Build history of the part. All positions in model axes, mm. A direction names the side the tool comes from. Give positions to 0.01 mm unless a question says otherwise; leave off trailing zeros. Write each loop counter-clockwise with the first axis right and the second up, starting at its lowest first coordinate (ties: lowest second). Pieces come first, ordered by that corner, then holes.
from build123d import *

# Parameters (mm, degrees)
ESQUISSE1_W        = 212
ESQUISSE1_H        = 75.3
ESQUISSE1_R        = 2
ESQUISSE1_W_2      = 5
ESQUISSE1_H_2      = 5
BOSS_EXTRU_1_DEPTH = 5


with BuildPart() as part:
    # Esquisse1 → Boss.-Extru.1 (new body)
    with BuildSketch(Plane.XY):
        with Locations((106, 0)):
            Rectangle(ESQUISSE1_W, ESQUISSE1_H)
        with Locations((30, 0)):
            Circle(ESQUISSE1_R, mode=Mode.SUBTRACT)
        with Locations((80, 0)):
            Circle(ESQUISSE1_R, mode=Mode.SUBTRACT)
        with Locations((82, 33.15)):
            Circle(ESQUISSE1_R, mode=Mode.SUBTRACT)
        with Locations((167, 33.15)):
            Circle(ESQUISSE1_R, mode=Mode.SUBTRACT)
        with Locations(Location((167, -33.15, 0), (0, 0, 90))):
            Circle(ESQUISSE1_R, mode=Mode.SUBTRACT)
        with Locations(Location((82, -33.15, 0), (0, 0, 90))):
            Circle(ESQUISSE1_R, mode=Mode.SUBTRACT)
        with Locations((74.5, 33.15)):
            Rectangle(ESQUISSE1_W_2, ESQUISSE1_H_2, mode=Mode.SUBTRACT)
        with Locations((89.5, 33.15)):
            Rectangle(ESQUISSE1_W_2, ESQUISSE1_H_2, mode=Mode.SUBTRACT)
        with Locations((159.5, 33.15)):
            Rectangle(ESQUISSE1_W_2, ESQUISSE1_H_2, mode=Mode.SUBTRACT)
        with Locations((174.5, 33.15)):
            Rectangle(ESQUISSE1_W_2, ESQUISSE1_H_2, mode=Mode.SUBTRACT)
        with Locations((159.5, -33.15)):
            Rectangle(ESQUISSE1_W_2, ESQUISSE1_H_2, mode=Mode.SUBTRACT)
        with Locations((174.5, -33.15)):
            Rectangle(ESQUISSE1_W_2, ESQUISSE1_H_2, mode=Mode.SUBTRACT)
        with Locations((74.5, -33.15)):
            Rectangle(ESQUISSE1_W_2, ESQUISSE1_H_2, mode=Mode.SUBTRACT)
        with Locations((89.5, -33.15)):
            Rectangle(ESQUISSE1_W_2, ESQUISSE1_H_2, mode=Mode.SUBTRACT)
    extrude(amount=BOSS_EXTRU_1_DEPTH)


solid = part.part
(1) Saw through at B-B, the plane y = 33.15. List the corners of the cut face in (x, z), plus the area to 3 significant figures.
(2) Saw through at D-D, the plane z = 4.2. Give the number of separate pieces and of enclosed holes in the cut face, plus the area to 3 significant figures.
(3) Mould opens along Y. For faces 1 (the face through (212, -1, 2)), 2 (the face through (159, -35.65, 2)) say: +Y half, -Y half, draft (parallel to the pull), parting line (faces both ways), or undercut.
(4) Probe line 1 (Y direction, x = 75, z = 4); line 2 (Y direction, x = 30, z = 1.85); line 3 (Y direction, x = 78.5, z = 4.3). List the from-to ranges inside material, lowest first.
(5) Drop a flat-ended pin along its axis: pin 1 (3.5 mm diameter, centred on x = 82, y = 33.15, fed in from -Z). Give the stop position or say it passes through.
(6) 3-axis set-ups, long thin cutter, end or side, ignore diameter. For faces 3 (the face through (0, -1, 2)), 4 (the face through (172, 33, 2)): which of +Z, -Z, +X, -X, +Y, -Y reach the whole face in a straight line?
(7) Saw through at A-A, the plane x = 30. List the corners of the cut face in (y, z).
(8) Saw through at C-C, the plane x = 167. List the corners of the cut face in (y, z).
Computed values:
1. outline: (0, 0) - (72, 0) - (72, 5) - (0, 5) - close; (77, 0) - (80, 0) - (80, 5) - (77, 5) - close; (84, 0) - (87, 0) - (87, 5) - (84, 5) - close; (92, 0) - (157, 0) - (157, 5) - (92, 5) - close; (162, 0) - (165, 0) - (165, 5) - (162, 5) - close; (169, 0) - (172, 0) - (172, 5) - (169, 5) - close; (177, 0) - (212, 0) - (212, 5) - (177, 5) - close
1. area: 920 mm2
2. separate pieces: 1
2. enclosed holes: 14
2. area: 15,700 mm2
3. face 1: draft
3. face 2: undercut
4. line 1: y = -37.65 to -35.65, -30.65 to 30.65, 35.65 to 37.65
4. line 2: y = -37.65 to -2, 2 to 37.65
4. line 3: y = -37.65 to -1.32, 1.32 to 37.65
5. pin 1: passes through
6. face 3: +Z, -Z, -X, +Y, -Y
6. face 4: +Z, -Z
7. outline: (-37.65, 0) - (-2, 0) - (-2, 5) - (-37.65, 5) - close; (2, 0) - (37.65, 0) - (37.65, 5) - (2, 5) - close
8. outline: (-37.65, 0) - (-35.15, 0) - (-35.15, 5) - (-37.65, 5) - close; (-31.15, 0) - (31.15, 0) - (31.15, 5) - (-31.15, 5) - close; (35.15, 0) - (37.65, 0) - (37.65, 5) - (35.15, 5) - close
